```python
from build123d import *

# Parameters (mm, degrees)
F0_R     = 57.15
F1_DEPTH = 76.2
F2_R     = 50.8
F3_DEPTH = 63.5
F4_R     = 6.35
F4_R_2   = 5.08
F5_DEPTH = 1524


# Not quite as in the source:
# - a fillet or chamfer that OpenCascade refuses, or shapes differently, is made with other operations: its cross-section is extruded or revolved along the edge and cut away or added


with BuildPart() as f1:
    # F0 (on Top) → F1 (new body)
    with BuildSketch(Plane.XY):
        Circle(F0_R)
    extrude(amount=F1_DEPTH)

    # F2 (on face) → F3 (cut)
    with BuildSketch(Plane.XY.offset(76.2)):
        Circle(F2_R)
    extrude(amount=-F3_DEPTH, mode=Mode.SUBTRACT)

    # F4 (on face) → F5 (join)
    with BuildSketch(Plane.XY.offset(12.7)):
        Circle(F4_R)
        Circle(F4_R_2, mode=Mode.SUBTRACT)
    extrude(amount=F5_DEPTH)

    # F6: chamfer of 2.54 on 1 edges, made by hand

    # F6_s1 → F6_t2 (revolve, cut)
    with BuildSketch(Plane.XZ):
        Polygon((6.35, 1534.16), (3.81, 1536.7), (6.35, 1536.7), align=None)
    revolve(axis=Axis((0, 0, 1536.7), (0, 0, 1)), mode=Mode.SUBTRACT)


solid = f1.part
```
Input: part model. Units: mm. Frame: model coordinates. Coordinates: 2 decimals unless noted, no trailing zeros. Order: outer loops, then holes, each group sorted by start corner. A loop starts at its lowest first (then second) coordinate and runs counter-clockwise, first axis right, second up. Notation, with made-up numbers: (3, 65.5) - (13, 65.5) arc R28 ccw to (13, 98.5) - close; hole circle Ø5 at (64.5, 0.5). An arc over 180 degrees is marked (long way). Return JSON: item names as keys, results as strings.
Q1. First-contact query: pin 1 (3 mm diameter, centred on x = -15, y = -23.5, fed in from +Z); pin 2 (13 mm diameter, centred on x = 0, y = 0, fed in from +Z). Flat tips, straight axial feed; report the tip coordinate or a pass-through.
The answers:
{"pin 1": "stops at z = 12.7", "pin 2": "stops at z = 1535.43"}
Q2. Ray query, probe 1 along Y at (x, z) = (0, 44); probe 2 along Y at (x, z) = (0, 862); probe 3 along Z at (x, y) = (30, 7). Return the intervals inside material, ascending.
The answers:
{"probe 1": "y = -57.15 to -50.8, -6.35 to -5.08, 5.08 to 6.35, 50.8 to 57.15", "probe 2": "y = -6.35 to -5.08, 5.08 to 6.35", "probe 3": "z = 0 to 12.7"}
Q3. Cut plane B-B (x = -36). Return loops of the section in (y, z).
The answers:
{"outline": "(-44.39, 0) - (44.39, 0) - (44.39, 76.2) - (35.84, 76.2) - (35.84, 12.7) - (-35.84, 12.7) - (-35.84, 76.2) - (-44.39, 76.2) - close"}
Q4. Draft query along X for faces 1 (the cylindrical face through (-57.095, 2.513, 37.567)), 2 (the flat face through (11, 1, 12.7)), 3 (the cylindrical face through (-11.012, -49.592, 44.894)), 4 (the flat face through (-38, -34, 76.2)). Return one class per face: +X half, -X half, draft (parallel to the pull), parting line (faces both ways), or undercut.
The answers:
{"face 1": "parting line", "face 2": "undercut", "face 3": "undercut", "face 4": "draft"}
Q5. Cut plane C-C (z = 286.5). Return loops of the section in (x, y), then the cut area to 3 significant figures.
The answers:
{"outline": "circle Ø12.7 at (0, 0); hole circle Ø10.16 at (0, 0)", "area": "45.6 mm2"}
Q6. Cut plane A-A (y = 21). Return loops of the section in (x, z).
The answers:
{"outline": "(-53.15, 0) - (53.15, 0) - (53.15, 76.2) - (46.26, 76.2) - (46.26, 12.7) - (-46.26, 12.7) - (-46.26, 76.2) - (-53.15, 76.2) - close"}
